Verification items for this drawing (mm, ordinates from the low corner). Round coordinates to 2 decimals unless told otherwise and drop trailing zeros. Write each loop counter-clockwise with the first axis right and the second up, starting at its lowest first coordinate (ties: lowest second). Pieces come first, ordered by that corner, then holes. Notation, with made-up numbers: M 76.5,-30 L 88.5,-30 A25 cw 88.5,0 Z; hole C 40.25,14.25 d9. An arc over 180 degrees is marked long. One line per question, with ' | ' between items. Start each with the question number.
Q1. Thickness scan on line 1 along Y through (x, z) = (2, 1.15); line 2 along X through (y, z) = (2.75, 1); line 3 along X through (y, z) = (9.75, 0.35). Record the ranges inside material, lowest first. Write a range as from..to.
Q2. Cross-section at D-D (x = 15.5). Record the boundary of the cut face in (y, z), then the cut area to 3 significant figures.
Q3. Cross-section at C-C (z = 0.9). Record the boundary of the cut face in (x, y).
Q4. Cross-section at A-A (y = 2). Record the boundary of the cut face in (x, z).
Q5. Cross-section at B-B (x = 22). Record the boundary of the cut face in (y, z).
Q6. Release check for a two-part mould opening along X. For the marked faces 1 and 2 record: released by +X, released by -X, zero draft, split by the parting line, or undercut.
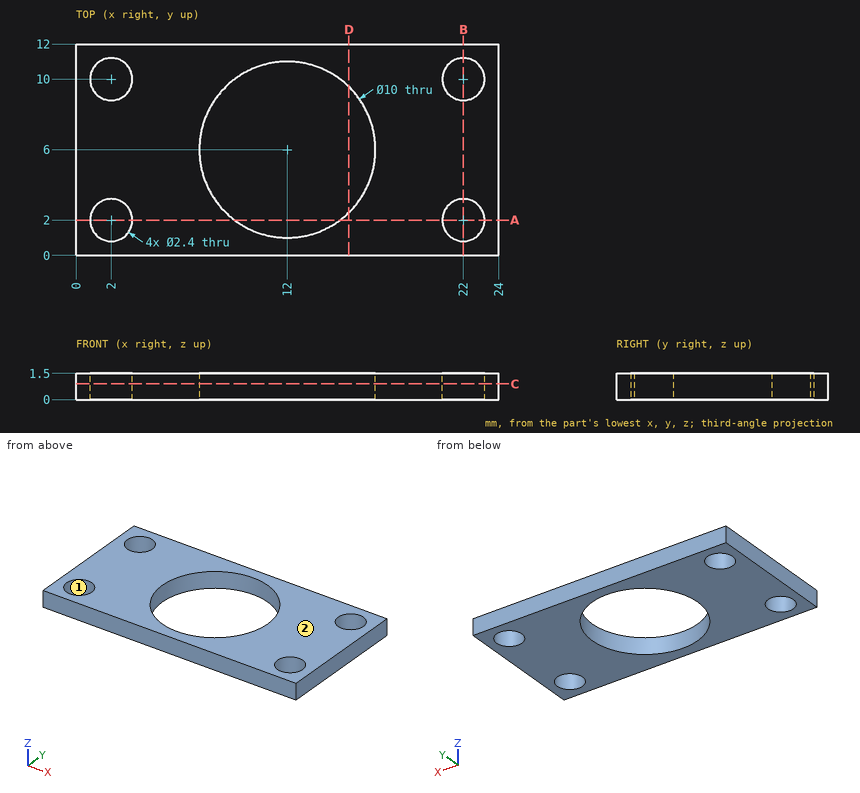
Determined:
1) line 1: y = 0..0.8, 3.2..8.8, 11.2..12 | line 2: x = 0..1.06, 2.94..8.2, 15.8..21.06, 22.94..24 | line 3: x = 0..0.83, 3.17..8.69, 15.31..20.83, 23.17..24
2) outline: M 0,0 L 2.43,0 L 2.43,1.5 L 0,1.5 Z; M 9.57,0 L 12,0 L 12,1.5 L 9.57,1.5 Z | area: 7.29 mm²
3) outline: M 0,0 L 24,0 L 24,12 L 0,12 Z; hole C 2,2 d2.4; hole C 2,10 d2.4; hole C 12,6 d10; hole C 22,2 d2.4; hole C 22,10 d2.4
4) outline: M 0,0 L 0.8,0 L 0.8,1.5 L 0,1.5 Z; M 3.2,0 L 9,0 L 9,1.5 L 3.2,1.5 Z; M 15,0 L 20.8,0 L 20.8,1.5 L 15,1.5 Z; M 23.2,0 L 24,0 L 24,1.5 L 23.2,1.5 Z
5) outline: M 0,0 L 0.8,0 L 0.8,1.5 L 0,1.5 Z; M 3.2,0 L 8.8,0 L 8.8,1.5 L 3.2,1.5 Z; M 11.2,0 L 12,0 L 12,1.5 L 11.2,1.5 Z
6) face 1: undercut | face 2: zero draft
